Answer from the drawing. Dimensions are ordinates in mm from the lowest x, y and z of the part. A direction names the side the tool comes from. Coordinates: 2 decimals unless noted, no trailing zeros. Order: outer loops, then holes, each group sorted by start corner. A loop starts at its lowest first (then second) coordinate and runs counter-clockwise, first axis right, second up. Notation, with made-up numbers: (19.5, 78) -> (27.5, 78) arc R23 cw to (27.5, 111) -> close; hole circle Ø4 at (74, -39.75). An arc over 180 degrees is marked (long way). Answer in a Markdown table with one row per item.
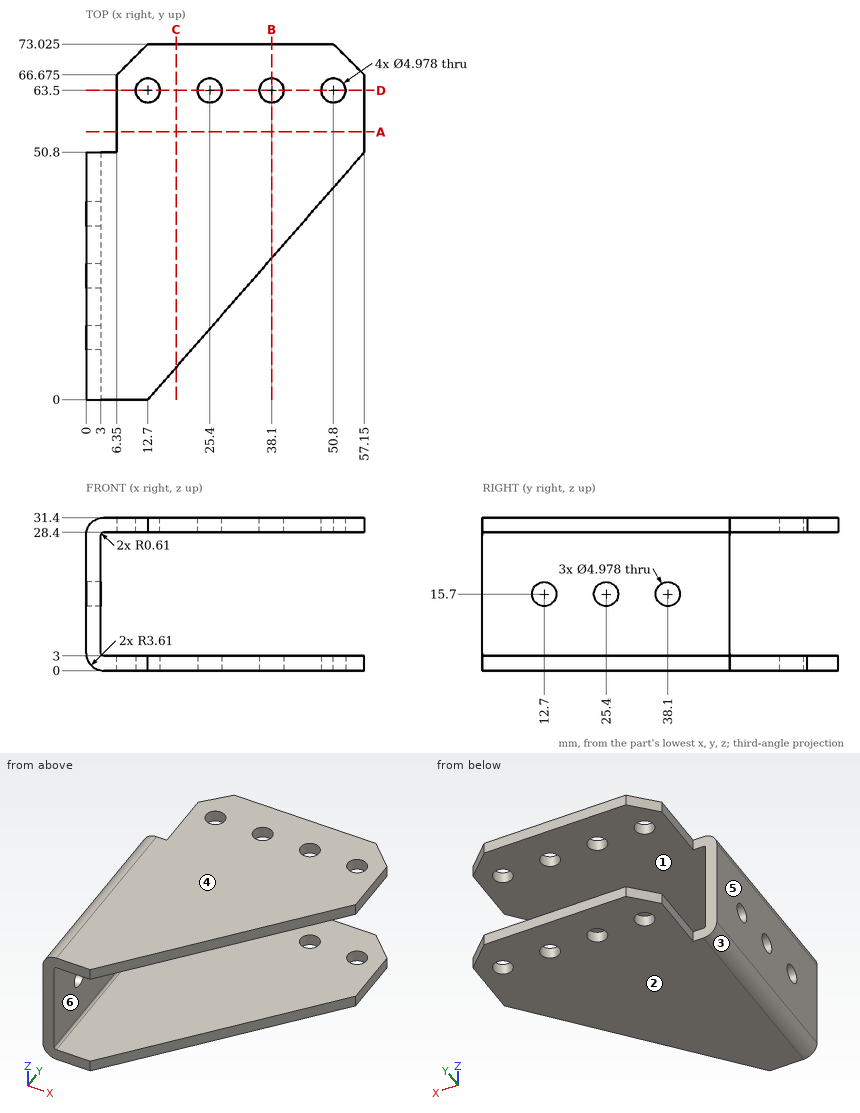
(1) A cutting plane is placed at C-C, the plane x = 18.5. Determine the outline of the cut face in (y, z) (1 decimal).
Check values:
| item | result |
|---|---|
| outline | (6.6, 0) -> (73, 0) -> (73, 3) -> (6.6, 3) -> close; (6.6, 28.4) -> (73, 28.4) -> (73, 31.4) -> (6.6, 31.4) -> close |
(2) Which of the six approach directions +Z, -Z, +X, -X, +Y, -Y give full straight-line access (tool end or side, diameter ignored) to the marked faces 1 and 2?
Check values:
| item | result |
|---|---|
| face 1 | +X, +Y, -Y |
| face 2 | -Z, +X, -X, +Y, -Y |
(3) A cutting plane is placed at D-D, the plane y = 63.5. Count the separate pieces of the cut face and the enclosed holes in it, then the cut area to 3 significant figures.
Check values:
| item | result |
|---|---|
| separate pieces | 10 |
| enclosed holes | 0 |
| area | 185 mm² |
(4) For a pull along Z with two mould halves and no side action, classify the marked faces 3, 4, 5 and 6 as released by +Z, released by -Z, zero draft, split by the parting line, or undercut.
Check values:
| item | result |
|---|---|
| face 3 | released by -Z |
| face 4 | released by +Z |
| face 5 | zero draft |
| face 6 | undercut |
(5) A cutting plane is placed at A-A, the plane y = 55. Determine the outline of the cut face in (x, z), then the cut area to 3 significant figures.
Check values:
| item | result |
|---|---|
| outline | (6.35, 0) -> (57.15, 0) -> (57.15, 3) -> (6.35, 3) -> close; (6.35, 28.4) -> (57.15, 28.4) -> (57.15, 31.4) -> (6.35, 31.4) -> close |
| area | 305 mm² |
(6) Flat-ended cylindrical pins translate along their axes: pin 1 (2.5 mm diameter, centred on y = 60, z = 30.5, fed in from -X); pin 2 (10 mm diameter, centred on y = 33, z = 27, fed in from +X) (1 decimal); pin 3 (3 mm diameter, centred on x = 3.5, z = 17, fed in from +Y). Find the tip coordinate at first contact, or state that the pin passes through.
Check values:
| item | result |
|---|---|
| pin 1 | x = 6.35 |
| pin 2 | x = 45.8 |
| pin 3 | y = 50.8 |
(7) A cutting plane is placed at B-B, the plane x = 38.1. Determine the outline of the cut face in (y, z) (1 decimal), then the cut area to 3 significant figures.
Check values:
| item | result |
|---|---|
| outline | (29, 0) -> (61, 0) -> (61, 3) -> (29, 3) -> close; (29, 28.4) -> (61, 28.4) -> (61, 31.4) -> (29, 31.4) -> close; (66, 0) -> (73, 0) -> (73, 3) -> (66, 3) -> close; (66, 28.4) -> (73, 28.4) -> (73, 31.4) -> (66, 31.4) -> close |
| area | 234 mm² |
(8) Find the intervals of material crossed by line 1 along X through (y, z) = (63.5, 30.75); line 2 along X through (y, z) = (63, 1); line 3 along Z through (x, y) = (6.5, 40), in increasing order. Write a range as from..to.
Check values:
| item | result |
|---|---|
| line 1 | 6.35..10.21, 15.19..22.91, 27.89..35.61, 40.59..48.31, 53.29..57.15 |
| line 2 | 6.35..10.26, 15.14..22.96, 27.84..35.66, 40.54..48.36, 53.24..57.15 |
| line 3 | 0..3, 28.4..31.4 |
